The model under review builds one solid part; all positions refer to its coordinate system, in mm. A direction names the side the tool comes from. Give positions to 0.01 mm unless a question says otherwise; leave off trailing zeros. Order: outer loops, then holes, each group sorted by start corner. A loop starts at its lowest first (then second) coordinate and runs counter-clockwise, first axis right, second up. Notation, with made-up numbers: (17.5, 74.5) - (73.5, 74.5) arc R29 cw to (73.5, 104.5) - close; hole circle Ø11 at (23.5, 66). An arc over 180 degrees is marked (long way). Answer as CSV lines item,"result". Start each with the question number.
from build123d import *

# Parameters (mm, degrees)
SKETCH1_W           = 50
SKETCH1_H           = 50
BOSS_EXTRUDE1_DEPTH = 1.6
SKETCH2_R           = 1.6
CUT_EXTRUDE1_DEPTH  = 2.6
FILLET1_R           = 1
SKETCH3_W           = 2.54
SKETCH3_H           = 42
SKETCH3_H_2         = 33
BOSS_EXTRUDE2_DEPTH = 8


with BuildPart() as part:
    # Sketch1 → Boss-Extrude1 (new body)
    with BuildSketch(Plane(origin=(0, 0, 0), x_dir=(1, 0, 0), z_dir=(0, 1, 0))):
        Rectangle(SKETCH1_W, SKETCH1_H)
    extrude(amount=BOSS_EXTRUDE1_DEPTH)

    # Sketch2 → Cut-Extrude1 (cut, through all)
    with BuildSketch(Plane(origin=(0, 1.6, 0), x_dir=(1, 0, 0), z_dir=(0, 1, 0))):
        with Locations((-13, -13)):
            Circle(SKETCH2_R)
        with Locations((13, 13)):
            Circle(SKETCH2_R)
    extrude(amount=-CUT_EXTRUDE1_DEPTH, mode=Mode.SUBTRACT)

    # Fillet1
    fillet1_edges = [part.edges().sort_by_distance(p)[0] for p in [
        (-25, 0.8, -25),
        (25, 0.8, -25),
        (25, 0.8, 25),
        (-25, 0.8, 25),
    ]]
    fillet(fillet1_edges, radius=FILLET1_R)

    # Sketch3 → Boss-Extrude2 (add)
    with BuildSketch(Plane(origin=(0, 1.6, 0), x_dir=(1, 0, 0), z_dir=(0, 1, 0))):
        with Locations((-23.73, 0)):
            Rectangle(SKETCH3_W, SKETCH3_H)
        with Locations((23.73, 4.5)):
            Rectangle(SKETCH3_W, SKETCH3_H_2)
    extrude(amount=BOSS_EXTRUDE2_DEPTH)


solid = part.part
Item 1: Mouldability with a two-part tool opening along X and no side actions: class faces 4 (the face through (-25, 5, 0)), 5 (the face through (-24, 9.6, 0)), 6 (the face through (-22.46, 6, 0)), 7 (the face through (0, 1.6, 0)) as released by +X, released by -X, zero draft, split by the parting line, or undercut.
Item 2: Take a section at C-C on y = 3. Write out the cut boundary in (x, z), and give its area (4 significant figures).
Item 3: Take a section at D-D on z = 2. Write out the cut boundary in (x, y).
Item 4: Machinability: for faces 1 (the face through (22.46, 6, -4)), 2 (the face through (-24, 6, -21)), 3 (the face through (-24, 6, 21)), which of the approach directions +Z, -Z, +X, -X, +Y, -Y give a long, thin tool a straight path to every point of the face, cutting with its end or side? Answer none if there is none.
Item 5: Take a section at B-B on z = -13. Write out the cut boundary in (x, y).
Item 6: For line 1 along X through (y, z) = (7, -9); line 2 along Z through (x, y) = (13, 0.8); line 3 along Z through (x, y) = (-13, 0.9), list the stretches that pass through material, from the lowest coordinate up.
Item 7: Take a section at A-A on x = 13. Write out the cut boundary in (y, z), and give its area (3 significant figures).
Item 8: Clearance check with flat-ended pins moving along their axes: pin 1 (2 mm diameter, centred on x = 24.5, y = 7.5, fed in from +Z); pin 2 (1.9 mm diameter, centred on x = 13, z = -13, fed in from +Y); pin 3 (3 mm diameter, centred on x = -16, z = -6.5, fed in from +Y); pin 4 (1 mm diameter, centred on y = 6, z = 17, fed in from +X). State where each tip first meets the part, or that it passes through.
Data:
1,face 4,"released by -X"
1,face 5,"zero draft"
1,face 6,"undercut"
1,face 7,"undercut"
2,outline,"(-25, -21) - (-22.46, -21) - (-22.46, 21) - (-25, 21) - close; (22.46, -21) - (25, -21) - (25, 12) - (22.46, 12) - close"
2,area,"190.5 mm^2"
3,outline,"(-25, 0) - (25, 0) - (25, 9.6) - (22.46, 9.6) - (22.46, 1.6) - (-22.46, 1.6) - (-22.46, 9.6) - (-25, 9.6) - close"
4,face 1,"+Z, -Z, +Y"
4,face 2,"-Z, +X, -X, +Y"
4,face 3,"+Z, +X, -X, +Y"
5,outline,"(-25, 0) - (11.4, 0) - (11.4, 1.6) - (-22.46, 1.6) - (-22.46, 9.6) - (-25, 9.6) - close; (14.6, 0) - (25, 0) - (25, 9.6) - (22.46, 9.6) - (22.46, 1.6) - (14.6, 1.6) - close"
6,line 1,"x = -25 to -22.46, 22.46 to 25"
6,line 2,"z = -25 to -14.6, -11.4 to 25"
6,line 3,"z = -25 to 11.4, 14.6 to 25"
7,outline,"(0, -25) - (1.6, -25) - (1.6, -14.6) - (0, -14.6) - close; (0, -11.4) - (1.6, -11.4) - (1.6, 25) - (0, 25) - close"
7,area,"74.9 mm^2"
8,pin 1,"stops at z = 12"
8,pin 2,"passes through"
8,pin 3,"stops at y = 1.6"
8,pin 4,"stops at x = -22.46"
